```python
from build123d import *

# Parameters (mm, degrees)
F1_DEPTH = 152.4
F2_DEPTH = 50.8
F4_DEPTH = 5.08


with BuildPart() as f1:
    # F0 (on Top) → F1 (new body)
    with BuildSketch(Plane.XY):
        Polygon((-38.839806, 38.839806), (-38.839806, -38.839806), (7.116021, -38.839806), (7.116021, 54.005228), align=None)
    extrude(amount=F1_DEPTH)

    # F0 (on Top) → F2 (join)
    with BuildSketch(Plane.XY):
        Polygon((7.116021, 54.005228), (7.116021, -38.839806), (38.839806, -38.839806), (88.813685, -38.839806), (38.839806, 64.474076), align=None)
    extrude(amount=F2_DEPTH)

    # F3 (on face) → F4 (join)
    with BuildSketch(Plane.XY.offset(152.4)):
        Polygon((5.012183, -36.509417), (5.012183, 51.268544), (-1.17696, 51.268544), (-36.934808, 39.468455), (-36.934808, -36.509417), align=None)
    extrude(amount=F4_DEPTH)


solid = f1.part
```
Geometry: final body of the model. Coordinates: model frame, mm. A direction names the side the tool comes from. Coordinates: 2 decimals unless noted, no trailing zeros. Loops run counter-clockwise (first coordinate to the right, second up) from the corner with the lowest first, then second, coordinate; pieces in that order, holes last. Notation, with made-up numbers: M 75,28 L 116,28 A16 ccw 116,48 Z; hole C 20.25,6.5 d4. An arc over 180 degrees is marked long. Put each result on its own line as item: value.
(1) Cut plane C-C on z = 132. Return the cut outline in (x, y).
Answer sheet:
outline: M -38.84,-38.84 L 7.12,-38.84 L 7.12,54.01 L -38.84,38.84 Z
(2) Cut plane B-B on y = -1.5. Return the cut outline in (x, z).
Answer sheet:
outline: M -38.84,0 L 70.75,0 L 70.75,50.8 L 7.12,50.8 L 7.12,152.4 L 5.01,152.4 L 5.01,157.48 L -36.93,157.48 L -36.93,152.4 L -38.84,152.4 Z
(3) Cut plane A-A on x = -21. Return the cut outline in (y, z).
Answer sheet:
outline: M -38.84,0 L 44.73,0 L 44.73,157.48 L -36.51,157.48 L -36.51,152.4 L -38.84,152.4 Z
(4) Cut plane D-D on y = 27. Return the cut outline in (x, z).
Answer sheet:
outline: M -38.84,0 L 56.97,0 L 56.97,50.8 L 7.12,50.8 L 7.12,152.4 L 5.01,152.4 L 5.01,157.48 L -36.93,157.48 L -36.93,152.4 L -38.84,152.4 Z
(5) Material intervals for probe 1 along X at (y, z) = (-4, 146); probe 2 along Z at (x, y) = (28.5, -6.5); probe 3 along Y at (x, z) = (-31, 113), sorted ascending.
Answer sheet:
probe 1: x = -38.84 to 7.12
probe 2: z = 0 to 50.8
probe 3: y = -38.84 to 41.43
(6) First-contact query: pin 1 (4 mm diameter, centred on y = 9.5, z = 66, fed in from +X); pin 2 (2.5 mm diameter, centred on y = 20.5, z = 156, fed in from +X); pin 3 (10 mm diameter, centred on x = 34, y = 30.5, fed in from +Z). Flat tips, straight axial feed; report the tip coordinate or a pass-through.
Answer sheet:
pin 1: stops at x = 7.12
pin 2: stops at x = 5.01
pin 3: stops at z = 50.8
(7) Access query for faces 1 (the face through (2, 51.269, 155)), 2 (the face through (-16, -36.509, 155)), 3 (the face through (7.116, 7, 101)). Directions: +Z, -Z, +X, -X, +Y, -Y. A direction counts if a zero-diameter tool reaches every point of the face in a straight line with its end or side. Return the directions, or none.
Answer sheet:
face 1: +Z, +X, -X, +Y
face 2: +Z, +X, -X, -Y
face 3: +Z, +X, +Y, -Y
